from build123d import *

# Parameters (mm, degrees)
SKETCH_1_W          = 22
SKETCH_1_H          = 76
EXTRUDE_1_DEPTH     = 50
SKETCH_5_W          = 20
SKETCH_5_H          = 42
SKETCH_5_W_2        = 12
CUT_EXTRUDE_1_DEPTH = 10
SKETCH_2_R          = 1.6
CUT_EXTRUDE_2_DEPTH = 10
SKETCH_3_R          = 1.6
CUT_EXTRUDE_3_DEPTH = 10
SKETCH_4_R          = 1.587
CUT_EXTRUDE_4_DEPTH = 10


with BuildPart() as part:
    # 草图1 → 凸台-拉伸1 (new body)
    with BuildSketch(Plane(origin=(0, 0, 0), x_dir=(1, 0, 0), z_dir=(0, 1, 0))):
        Polygon((0, 0), (69, 0), (69, 2), (51, 2), (51, 78), (69, 78), (69, 80), (0, 80), align=None)
        with Locations((14, 40)):
            Rectangle(SKETCH_1_W, SKETCH_1_H, mode=Mode.SUBTRACT)
        with Locations((38, 40)):
            Rectangle(SKETCH_1_W, SKETCH_1_H, mode=Mode.SUBTRACT)
    extrude(amount=EXTRUDE_1_DEPTH)

    # 草图5 → 切除-拉伸1 (cut)
    with BuildSketch(Plane.XY):
        with Locations((13, 25)):
            Rectangle(SKETCH_5_W, SKETCH_5_H)
        with Locations((38, 25)):
            Rectangle(SKETCH_5_W, SKETCH_5_H)
        with Locations((59, 25)):
            Rectangle(SKETCH_5_W_2, SKETCH_5_H)
    cut_extrude_1 = extrude(amount=-CUT_EXTRUDE_1_DEPTH, mode=Mode.SUBTRACT)

    # 镜向1: 切除-拉伸1 across plane
    add(cut_extrude_1.mirror(Plane.XY.offset(-40)), mode=Mode.SUBTRACT)

    # 草图2 → 切除-拉伸2 (cut)
    with BuildSketch(Plane(origin=(51, 0, 0), x_dir=(0, 0, -1), z_dir=(1, 0, 0))):
        with Locations((40, 33.85)):
            Circle(SKETCH_2_R)
        with Locations((40, 16.15)):
            Circle(SKETCH_2_R)
    extrude(amount=-CUT_EXTRUDE_2_DEPTH, mode=Mode.SUBTRACT)

    # 草图3 → 切除-拉伸3 (cut)
    with BuildSketch(Plane(origin=(27, 0, 0), x_dir=(0, 0, -1), z_dir=(1, 0, 0))):
        with Locations((15.046260159, 7.75)):
            Circle(SKETCH_3_R)
        with Locations((65.046260159, 7.75)):
            Circle(SKETCH_3_R)
        with Locations((15.046260159, 42.25)):
            Circle(SKETCH_3_R)
        with Locations((65.046260159, 42.25)):
            Circle(SKETCH_3_R)
    extrude(amount=-CUT_EXTRUDE_3_DEPTH, mode=Mode.SUBTRACT)

    # 草图4 → 切除-拉伸4 (cut)
    with BuildSketch(Plane(origin=(3, 0, 0), x_dir=(0, 0, -1), z_dir=(1, 0, 0))):
        with Locations((69.78201983, 5.121000004)):
            Circle(SKETCH_4_R)
        with Locations((9.78201983, 45.121000004)):
            Circle(SKETCH_4_R)
    extrude(amount=-CUT_EXTRUDE_4_DEPTH, mode=Mode.SUBTRACT)


solid = part.part
Read the model definition and answer for the solid it produces. Units are mm, in the model's axes. A direction names the side the tool comes from. Coordinates: 2 decimals unless noted, no trailing zeros. Loops run counter-clockwise (first coordinate to the right, second up) from the corner with the lowest first, then second, coordinate; pieces in that order, holes last. Notation, with made-up numbers: (25, 48.25) -> (29, 48.25) arc R18 cw to (29, 53.25) -> close; hole circle Ø6 at (17.5, 75). An arc over 180 degrees is marked (long way). Write item = value, one per line. Start each with the question number.
1) Find the intervals of material crossed by L1, parallel to X at y = 36, z = -26; L2, parallel to Z at x = 26, y = 42; L3, parallel to Y at x = 50.45, z = -40, in increasing order. Write a range as from..to.
2) The part is cut by section B-B, the plane x = 7.5. Determine the outline of the cut face in (y, z).
3) The part is cut by section D-D, the plane y = 7.75. State how many separate pieces and enclosed holes the cut face has, plus the area to 3 significant figures.
4) The part is cut by section C-C, the plane z = -75. Determine the outline of the cut face in (x, y).
5) Given P1, Ø5, axis at y = 19, z = -38, coming from the +X side, flat-ended and moving along its own axis, determine where the tip first touches the part or whether it passes through.
6) For faces 1 (the face through (26.01, 40.83, -15.78)), 2 (the face through (66, 25, -78)), 3 (the face through (49, 25, -39)), 4 (the face through (28, 25, -1)), determine the directions among +Z, -Z, +X, -X, +Y, -Y from which every point of the face is accessible in a straight line to the end or side of a thin tool.
7) The mould has two halves that part along X. Classify faces 5 (the face through (48, 25, -1)), 6 (the face through (50.01, 14.59, -39.65)), 7 (the face through (69, 25, -1)): pulls with the +X half, pulls with the -X half, needs draft (parallel to the pull), parting line crosses it, or undercut.
8) The part is cut by section A-A, the plane z = -40. Determine the outline of the cut face in (x, y), plus the area to 3 significant figures.
Result:
q1.L1 = 0..3, 25..27, 49..51
q1.L2 = -80..-66.63, -63.47..-16.63, -13.47..0
q1.L3 = 0..14.55, 17.75..32.25, 35.45..50
q2.outline = (0, -80) -> (4, -80) -> (4, -78) -> (0, -78) -> close; (0, -2) -> (4, -2) -> (4, 0) -> (0, 0) -> close; (46, -80) -> (50, -80) -> (50, -78) -> (46, -78) -> close; (46, -2) -> (50, -2) -> (50, 0) -> (46, 0) -> close
q3.separate_pieces = 7
q3.enclosed_holes = 0
q3.area = 587 mm²
q4.outline = (0, 0) -> (3, 0) -> (3, 50) -> (0, 50) -> close; (25, 0) -> (27, 0) -> (27, 50) -> (25, 50) -> close; (49, 0) -> (51, 0) -> (51, 50) -> (49, 50) -> close
q5.P1 = 51
q6.face_1 = none
q6.face_2 = +X, +Y, -Y
q6.face_3 = +Y, -Y
q6.face_4 = +Z, -Z
q7.face_5 = undercut
q7.face_6 = needs draft
q7.face_7 = pulls with the +X half
q8.outline = (0, 0) -> (3, 0) -> (3, 50) -> (0, 50) -> close; (25, 0) -> (27, 0) -> (27, 50) -> (25, 50) -> close; (49, 0) -> (51, 0) -> (51, 14.55) -> (49, 14.55) -> close; (49, 17.75) -> (51, 17.75) -> (51, 32.25) -> (49, 32.25) -> close; (49, 35.45) -> (51, 35.45) -> (51, 50) -> (49, 50) -> close
q8.area = 337 mm²
